Work out the finished part from the listing and answer in its coordinate system (mm). A direction names the side the tool comes from. Round coordinates to 2 decimals unless told otherwise and drop trailing zeros. Loops run counter-clockwise (first coordinate to the right, second up) from the corner with the lowest first, then second, coordinate; pieces in that order, holes last.
```python
from build123d import *

# Parameters (mm, degrees)
SZKIC1_W                      = 9.053278123
SZKIC1_H                      = 2.4000014
SZKIC1_R                      = 1.00000054
DODANIE_WYCI_GNI_CIE1_DEPTH   = 1.8
SZKIC1_W_2                    = 2.468942166
SZKIC1_H_2                    = 9.307035938
DODANIE_WYCI_GNI_CIE1_2_DEPTH = 1.8
SZKIC1_W_3                    = 8.953699963
SZKIC1_H_3                    = 3.54899108
SZKIC1_R_2                    = 1.10000034
DODANIE_WYCI_GNI_CIE1_3_DEPTH = 1.8
SZKIC2_R                      = 1.00000054
SZKIC2_R_2                    = 1.10000034
DODANIE_WYCI_GNI_CIE2_DEPTH   = 1.2
WYTNIJ_WYCI_GNI_CIE1_START    = -1.5
SZKIC3_W                      = 4.104918972
SZKIC3_H                      = 5
SZKIC3_R                      = 1.00000054
SZKIC3_W_2                    = 6
SZKIC3_H_2                    = 4.77449554
SZKIC3_R_2                    = 1.10000034
SZKIC3_H_3                    = 4.2000007
WYTNIJ_WYCI_GNI_CIE1_DEPTH    = 1.5
SZKIC7_W                      = 10
SZKIC7_H                      = 1.2
DODANIE_WYCI_GNI_CIE3_DEPTH   = 4
SZKIC8_W                      = 5.950377167
SZKIC8_H                      = 2
DODANIE_WYCI_GNI_CIE4_DEPTH   = 11
SZKIC9_W                      = 5.950377167
SZKIC9_H                      = 26.47425658
DODANIE_WYCI_GNI_CIE5_DEPTH   = 2
ZAOKR_GLENIE4_R               = 0.5


with BuildPart() as part:
    # Szkic1 → Dodanie-wyci_gni_cie1 (new body)
    with BuildSketch(Plane.XY.offset(158.832884642)):
        with Locations((-14.973320297, -21.27425588)):
            Rectangle(SZKIC1_W, SZKIC1_H)
        with Locations((-14.973320296, -21.27425588)):
            Circle(SZKIC1_R, mode=Mode.SUBTRACT)
    extrude(amount=DODANIE_WYCI_GNI_CIE1_DEPTH)



with BuildPart() as body_2:
    # Szkic1 → Dodanie-wyci_gni_cie1 2 (new body)
    with BuildSketch(Plane.XY.offset(158.832884642)):
        with Locations((8.247126613, -11.430282713)):
            Rectangle(SZKIC1_W_2, SZKIC1_H_2)
        with Locations((8.376678724, -10.97425616)):
            Circle(SZKIC1_R, mode=Mode.SUBTRACT)
    extrude(amount=DODANIE_WYCI_GNI_CIE1_2_DEPTH)


with BuildPart() as body_3:
    # Szkic1 → Dodanie-wyci_gni_cie1 3 (new body)
    with BuildSketch(Plane.XY.offset(158.832884642)):
        with Locations((-14.923531217, -1.77449554)):
            Rectangle(SZKIC1_W_3, SZKIC1_H_3)
        with Locations((-14.923531216, -1.77449554)):
            Circle(SZKIC1_R_2, mode=Mode.SUBTRACT)
    extrude(amount=DODANIE_WYCI_GNI_CIE1_3_DEPTH)


with BuildPart() as part_1:
    add(part.part)

    add(body_2.part)  # Dodanie-wyci_gni_cie2 merges body 2

    add(body_3.part)  # Dodanie-wyci_gni_cie2 merges body 3
    # Szkic2 → Dodanie-wyci_gni_cie2 (add)
    with BuildSketch(Plane.XY.offset(160.632884642)):
        Polygon((9.481597696, 0), (-19.400381198, 0), (-19.499959358, -22.47425658), (9.481597696, -22.47425658), align=None)
        with Locations((8.376678724, -10.97425616)):
            Circle(SZKIC2_R, mode=Mode.SUBTRACT)
        with Locations((-14.973320296, -21.27425588)):
            Circle(SZKIC2_R, mode=Mode.SUBTRACT)
        with Locations((-14.923531216, -1.77449554)):
            Circle(SZKIC2_R_2, mode=Mode.SUBTRACT)
    extrude(amount=DODANIE_WYCI_GNI_CIE2_DEPTH)

    # Szkic3 → Wytnij-wyci_gni_cie1 (cut)
    # profile 1 of 3: a face of its own
    with BuildSketch(Plane.XY.offset(161.832884642).offset(WYTNIJ_WYCI_GNI_CIE1_START)):
        with Locations((7.42913821, -10.97425616)):
            Rectangle(SZKIC3_W, SZKIC3_H)
        with Locations((8.376678724, -10.97425616)):
            Circle(SZKIC3_R, mode=Mode.SUBTRACT)
    # profile 2 of 3: a face of its own
    with BuildSketch(Plane.XY.offset(161.832884642).offset(WYTNIJ_WYCI_GNI_CIE1_START)):
        with Locations((-14.923531216, -2.38724777)):
            Rectangle(SZKIC3_W_2, SZKIC3_H_2)
        with Locations((-14.923531216, -1.77449554)):
            Circle(SZKIC3_R_2, mode=Mode.SUBTRACT)
    # profile 3 of 3: a face of its own
    with BuildSketch(Plane.XY.offset(161.832884642).offset(WYTNIJ_WYCI_GNI_CIE1_START)):
        with Locations((-14.973320296, -20.37425623)):
            Rectangle(SZKIC3_W_2, SZKIC3_H_3)
        with Locations((-14.973320296, -21.27425588)):
            Circle(SZKIC3_R, mode=Mode.SUBTRACT)
    extrude(amount=WYTNIJ_WYCI_GNI_CIE1_DEPTH, mode=Mode.SUBTRACT)

    # Szkic7 → Dodanie-wyci_gni_cie3 (add)
    with BuildSketch(Plane(origin=(0, 0, 0), x_dir=(1, 0, 0), z_dir=(0, 1, 0))):
        with Locations((4.481597696, -161.232884642)):
            Rectangle(SZKIC7_W, SZKIC7_H)
    extrude(amount=DODANIE_WYCI_GNI_CIE3_DEPTH)

    # Szkic8 → Dodanie-wyci_gni_cie4 (add)
    with BuildSketch(Plane.XY.offset(161.832884642)):
        with Locations((4.45678628, 3)):
            Rectangle(SZKIC8_W, SZKIC8_H)
        with Locations((4.45678628, -21.47425658)):
            Rectangle(SZKIC8_W, SZKIC8_H)
    extrude(amount=DODANIE_WYCI_GNI_CIE4_DEPTH)

    # Szkic9 → Dodanie-wyci_gni_cie5 (add)
    with BuildSketch(Plane.XY.offset(172.832884642)):
        with Locations((4.45678628, -9.23712829)):
            Rectangle(SZKIC9_W, SZKIC9_H)
    extrude(amount=DODANIE_WYCI_GNI_CIE5_DEPTH)

    # Zaokr_glenie4
    zaokr_glenie4_edges = [part_1.edges().sort_by_distance(p)[0] for p in [
        (-11.973320296, -20.37425623, 161.832884642),
        (-14.973320296, -18.27425588, 161.832884642),
        (-17.973320296, -20.37425623, 161.832884642),
        (-6.22096676, 0, 161.832884642),
        (-0.518402304, 2, 161.832884642),
        (0.481597696, 4, 161.832884642),
        (8.456786279, 4, 161.832884642),
        (7.431974863, 2, 167.332884642),
        (7.431974863, 4, 168.332884642),
        (1.481597696, 4, 168.332884642),
        (1.481597696, 2, 167.332884642),
        (8.456786279, -22.47425658, 161.832884642),
        (7.431974863, -22.47425658, 168.332884642),
        (7.431974863, -20.47425658, 167.332884642),
        (1.481597696, -22.47425658, 168.332884642),
        (7.431974863, -9.23712829, 172.832884642),
        (1.481597696, -9.23712829, 172.832884642),
        (7.431974863, -9.23712829, 174.832884642),
        (4.456786279, 4, 174.832884642),
        (1.481597696, -9.23712829, 174.832884642),
        (4.456786279, -22.47425658, 174.832884642),
        (9.481597696, -17.97425637, 161.832884642),
        (-19.450170278, -11.23712829, 161.832884642),
        (-18.736639827, -22.47425658, 161.832884642),
        (-18.661956207, 0, 161.832884642),
        (9.481597696, -2.23712808, 161.832884642),
        (-5.2458613, -22.47425658, 161.832884642),
        (7.42913821, -8.47425616, 161.832884642),
        (5.376678724, -10.97425616, 161.832884642),
        (7.42913821, -13.47425616, 161.832884642),
        (-17.923531216, -2.38724777, 161.832884642),
        (-14.923531216, -4.77449554, 161.832884642),
        (-11.923531216, -2.38724777, 161.832884642),
    ]]
    fillet(zaokr_glenie4_edges, radius=ZAOKR_GLENIE4_R)


solid = part_1.part
```
1. Which of the six approach directions +Z, -Z, +X, -X, +Y, -Y give full straight-line access (tool end or side, diameter ignored) to faces 1 (the face through (8.2, -9.8, 160.333)), 2 (the face through (1.482, -11, 174)), 3 (the face through (7, -13.474, 161))?
Answer key:
face 1: +X, -X
face 2: +Z, -X, +Y, -Y
face 3: +X
2. Find section A-A (z = 164.5). Write down the section's boundary in (x, y), then the cut area to 3 significant figures.
Answer key:
outline: (1.48, -21.97) arc R0.5 ccw to (1.98, -22.47) - (6.93, -22.47) arc R0.5 ccw to (7.43, -21.97) - (7.43, -20.97) arc R0.5 ccw to (6.93, -20.47) - (1.48, -20.47) - close; (1.48, 2.5) arc R0.5 ccw to (1.98, 2) - (6.93, 2) arc R0.5 ccw to (7.43, 2.5) - (7.43, 3.5) arc R0.5 ccw to (6.93, 4) - (1.98, 4) arc R0.5 ccw to (1.48, 3.5) - close
area: 23.4 mm2
3. Find section D-D (x = -11). Write down the section's boundary in (y, z), then the cut area to 3 significant figures.
Answer key:
outline: (-22.47, 158.83) - (-20.07, 158.83) - (-20.07, 160.63) - (-3.55, 160.63) - (-3.55, 158.83) - (0, 158.83) - (0, 161.33) arc R0.5 ccw to (-0.5, 161.83) - (-21.97, 161.83) arc R0.5 ccw to (-22.47, 161.33) - close
area: 37.6 mm2
4. Find section C-C (y = 0.5). Write down the section's boundary in (x, z), then the cut area to 3 significant figures.
Answer key:
outline: (-0.52, 160.63) - (9.48, 160.63) - (9.48, 161.33) arc R0.5 ccw to (8.98, 161.83) - (-0.02, 161.83) arc R0.5 ccw to (-0.52, 161.33) - close; (1.48, 173.33) arc R0.5 ccw to (1.98, 172.83) - (6.93, 172.83) arc R0.5 ccw to (7.43, 173.33) - (7.43, 174.33) arc R0.5 ccw to (6.93, 174.83) - (1.98, 174.83) arc R0.5 ccw to (1.48, 174.33) - close
area: 23.6 mm2
5. Consider probe 1 along Z at (x, y) = (3.5, -16); probe 2 along X at (y, z) = (-21, 169); probe 3 along Z at (x, y) = (-12.25, -14.75). Determine where each line is inside the solid, lowest interval first.
Answer key:
probe 1: z = 160.63 to 161.83, 172.83 to 174.83
probe 2: x = 1.48 to 7.43
probe 3: z = 160.63 to 161.83
6. Find section B-B (x = 2.75). Write down the section's boundary in (y, z), then the cut area to 3 significant figures.
Answer key:
outline: (-22.47, 160.63) - (4, 160.63) - (4, 174.33) arc R0.5 ccw to (3.5, 174.83) - (-21.97, 174.83) arc R0.5 ccw to (-22.47, 174.33) - close; hole (-20.47, 161.83) - (2, 161.83) - (2, 172.83) - (-20.47, 172.83) - close
area: 129 mm2
7. Determine the mould class of faces 4 (the face through (2.4, -22.474, 165.4)), 5 (the face through (7, -8.474, 161)), 6 (the face through (-16, -1, 158.833)) for opening direction Z: +Z half, -Z half, draft (parallel to the pull), parting line (faces both ways), or undercut.
Answer key:
face 4: draft
face 5: undercut
face 6: -Z half
8. Given pin 1 (1.4 mm diameter, centred on x = 8, z = 160, fed in from +Y); pin 2 (1.4 mm diameter, centred on y = -9.5, z = 160, fed in from -X); pin 3 (12 mm diameter, centred on x = -7.5, y = -9, fed in from -Z); pin 4 (6 mm diameter, centred on x = -12.5, z = 164.5, fed in from -Y), each flat-ended and moving along its own axis, determine where each tip first touches the part or whether it passes through.
Answer key:
pin 1: stops at y = 4
pin 2: stops at x = -19.44
pin 3: stops at z = 160.63
pin 4: stops at y = -22.42
